Can you work these out from the model? Positions are in its coordinate system, mm. Give positions to 0.01 mm unless a question says otherwise; leave off trailing zeros. Loops run counter-clockwise (first coordinate to the right, second up) from the corner with the lowest first, then second, coordinate; pieces in that order, holes last. Notation, with made-up numbers: (-21.75, 84) - (28.25, 84) arc R27 cw to (28.25, 101) - close; hole circle Ø8 at (47, 83). An arc over 180 degrees is marked (long way). Answer as a JSON object with one key per item and string values.
Solid Edge part; units mm, degrees
sketch "Sketch1" plane through (0, 0, 0) normal (0, -1, 0) x (1, 0, 0)
  line L0 (-65, -35) -> (65, -35)
  line L1 (65, -35) -> (65, 35)
  line L2 (65, 35) -> (-65, 35)
  line L3 (-65, 35) -> (-65, -35)
  dimension "D1" = 65
  dimension "D2" = 65
extrude "Ajout_matière_1" add sketch "Sketch1" along normal blind 3
sketch "Sketch2" plane through (0, -3, 0) normal (0, -1, 0) x (1, 0, 0)
  circle A0 centre (35, 0) radius 10
extrude "Enlèvement_matière_1" cut sketch "Sketch2" against normal blind 203.2796
sketch "Sketch3" plane through (0, -3, 0) normal (0, -1, 0) x (1, 0, 0)
  circle A0 centre (40, 20) radius 0.85
  circle A1 centre (15, 31) radius 1.55
  circle A2 centre (50, -20) radius 0.85
  circle A3 centre (61, -31) radius 1.55
  dimension "D1" = 40
  dimension "D2" = 50
extrude "Enlèvement_matière_2" cut sketch "Sketch3" against normal blind 33.5111
sketch "Sketch4" plane through (0, -3, 0) normal (0, -1, 0) x (1, 0, 0)
  line L0 (5, -32) -> (5, -38)
  line L1 (5, -38) -> (25, -38)
  line L2 (25, -38) -> (25, -32)
  line L3 (16.75, -32) -> (25, -32)
  line L4 (16.75, -29) -> (16.75, -32)
  line L5 (17.77, -29) -> (16.75, -29)
  line L6 (17.77, -26.2) -> (17.77, -29)
  line L7 (16.75, -26.2) -> (17.77, -26.2)
  line L8 (16.75, -24) -> (16.75, -26.2)
  line L9 (13.25, -24) -> (16.75, -24)
  line L10 (13.25, -26.2) -> (13.25, -24)
  line L11 (12.23, -26.2) -> (13.25, -26.2)
  line L12 (12.23, -29) -> (12.23, -26.2)
  line L13 (13.25, -29) -> (12.23, -29)
  line L14 (13.25, -32) -> (13.25, -29)
  line L15 (5, -32) -> (13.25, -32)
  dimension "D1" = 5
  dimension "D2" = 5
  dimension "D3" = 5
  dimension "D4" = 5
  dimension "D5" = 13.25
  dimension "D6" = 12.23
  dimension "D7" = 13.25
  dimension "D8" = 13.25
extrude "Cutout1" cut sketch "Sketch4" against normal blind 7.0408
mirror "Mirror1" about plane through (0, 0, 0) normal (1, 0, 0) of "Enlèvement_matière_2", "Enlèvement_matière_1", "Cutout1"
fillet "Round1" radius 20 2 edges at (-65, -1.5, 35) (65, -1.5, 35)
sketch "Sketch5" plane through (0, -3, 0) normal (0, -1, 0) x (1, 0, 0)
  circle A0 centre (0, 0) radius 5
extrude "Enlèvement_matière_5" cut sketch "Sketch5" against normal blind 16.0842
properties part number "06" material "MDF 3mm"
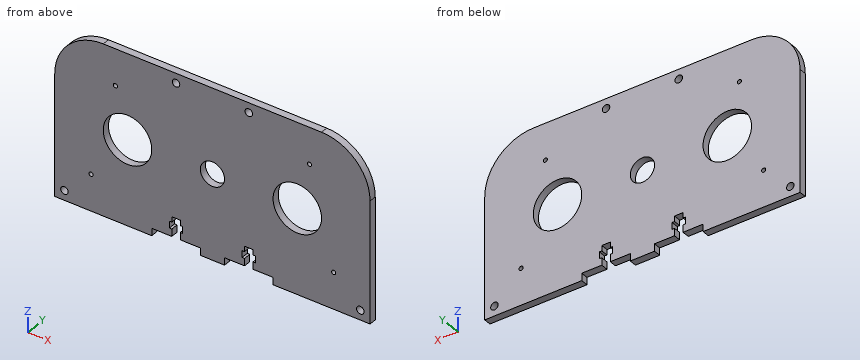
1) Imagine slicing it at D-D on x = -35. Write out the boundary of the cut face in (y, z).
Check sheet entries:
{"outline": "(-3, -35) - (0, -35) - (0, -10) - (-3, -10) - close; (-3, 10) - (0, 10) - (0, 35) - (-3, 35) - close"}
2) Imagine slicing it at C-C on z = 31. Write out the boundary of the cut face in (x, y), and give its area (3 significant figures).
Check sheet entries:
{"outline": "(-57, -3) - (-16.55, -3) - (-16.55, 0) - (-57, 0) - close; (-13.45, -3) - (13.45, -3) - (13.45, 0) - (-13.45, 0) - close; (16.55, -3) - (57, -3) - (57, 0) - (16.55, 0) - close", "area": "323 mm2"}
3) Imagine slicing it at B-B on z = 0. Write out the boundary of the cut face in (x, y), and give its area (3 significant figures).
Check sheet entries:
{"outline": "(-65, -3) - (-45, -3) - (-45, 0) - (-65, 0) - close; (-25, -3) - (-5, -3) - (-5, 0) - (-25, 0) - close; (5, -3) - (25, -3) - (25, 0) - (5, 0) - close; (45, -3) - (65, -3) - (65, 0) - (45, 0) - close", "area": "240 mm2"}
4) Imagine slicing it at A-A on x = -61. Write out the boundary of the cut face in (y, z).
Check sheet entries:
{"outline": "(-3, -35) - (0, -35) - (0, -32.55) - (-3, -32.55) - close; (-3, -29.45) - (0, -29.45) - (0, 27) - (-3, 27) - close"}
5) I'm going to push flat-ended pins straight in: P1, Ø12, axis at x = -48, z = -4.5, coming from the +Y side; P2, Ø1.5, axis at x = -15, y = -1.5, coming from the -Z side; P3, Ø1.1, axis at x = 12.5, y = -1, coming from the -Z side. Where does each tip first touch, or does it pass through?
Check sheet entries:
{"P1": "y = 0", "P2": "z = -24", "P3": "z = -32"}
6) I need wall thicknesses on L1, parallel to X at y = -2.1, z = -27; L2, parallel to X at y = -2.5, z = 0.5; L3, parallel to Z at x = -35.5, y = -1.75. Which ranges of each line are inside material? Lowest first, please.
Check sheet entries:
{"L1": "-65 to -17.77, -12.23 to 12.23, 17.77 to 65", "L2": "-65 to -44.99, -25.01 to -4.97, 4.97 to 25.01, 44.99 to 65", "L3": "-35 to -9.99, 9.99 to 35"}
